from build123d import *

# Parameters (mm, degrees)
SKETCH1_W          = 127
SKETCH1_H          = 6.35
SKETCH2_R          = 6.35
CUT_EXTRUDE1_DEPTH = 4.826


with BuildPart() as part:
    # Sketch1 → Revolve1 (revolve)
    with BuildSketch(Plane.XY, mode=Mode.PRIVATE) as revolve1_sk:
        with BuildLine():
            Line((127, 0), (127, 6.35))
            ThreePointArc((127, 6.35), (135.980256121, 10.069743879), (139.7, 19.05))
            Line((139.7, 19.05), (146.05, 19.05))
            ThreePointArc((146.05, 19.05), (140.470384182, 5.579615818), (127, 0))
        make_face()
        with Locations((63.5, 3.175)):
            Rectangle(SKETCH1_W, SKETCH1_H)
    revolve(revolve1_sk.sketch.rotate(Axis((0, 0, 0), (0, 1, 0)), 90), axis=Axis((0, 0, 0), (0, 1, 0)))

    # Sketch2 → Cut-Extrude1 (cut)
    with BuildSketch(Plane.XZ):
        with Locations(Location((0, 0, 0), (0, 0, 270))):
            Circle(SKETCH2_R)
    extrude(amount=-CUT_EXTRUDE1_DEPTH, mode=Mode.SUBTRACT)


solid = part.part
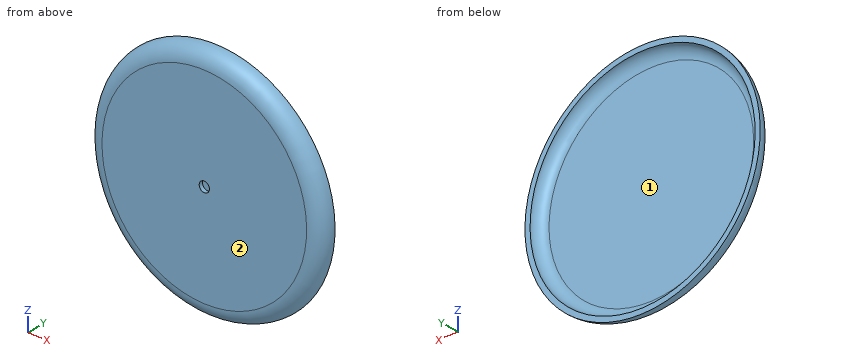
Part model, mm, in its own coordinate system. Face numbers are marked on the shaded views. Coordinates: 2 decimals unless noted, no trailing zeros. Order: outer loops, then holes, each group sorted by start corner. A loop starts at its lowest first (then second) coordinate and runs counter-clockwise, first axis right, second up. Notation, with made-up numbers: M 4.25,47 L 52.25,47 A24 cw 52.25,73 Z; hole C 54,54.5 d11. An arc over 180 degrees is marked long. One line per question, with ' | ' between items.
Q1. Slice it at C-C (y = 13.25). Give the cut face in (x, z).
A:
outline: C 0,0 d290.29; hole C 0,0 d276.6
Q2. Slice it at B-B (z = 0). Give the cut face in (x, y), and give its area (3 significant figures).
A:
outline: M -146.05,19.05 A19.05 ccw -127,0 L -6.35,0 L -6.35,4.83 L 6.35,4.83 L 6.35,0 L 127,0 A19.05 ccw 146.05,19.05 L 139.7,19.05 A12.7 cw 127,6.35 L -127,6.35 A12.7 cw -139.7,19.05 Z | area: 1,870 mm^2
Q3. Two-plate mould, pull along Z, no slides. Class the marked faces 1 and 2: +Z half, -Z half, draft (parallel to the pull), parting line (faces both ways), or undercut.
A:
face 1: undercut | face 2: draft
Q4. Slice it at A-A (x = 0). Give the cut face in (y, z), and give its area (3 significant figures).
A:
outline: M 0,-127 A19.05 ccw 19.05,-146.05 L 19.05,-139.7 A12.7 cw 6.35,-127 L 6.35,127 A12.7 cw 19.05,139.7 L 19.05,146.05 A19.05 ccw 0,127 L 0,6.35 L 4.83,6.35 L 4.83,-6.35 L 0,-6.35 Z | area: 1,870 mm^2
Q5. Pin check, flat tips, straight feed: P1, Ø10, axis at y = 3.5, z = -41, coming from the +X side; P2, Ø8, axis at y = 4, z = 63.5, coming from the +X side; P3, Ø1, axis at y = 2, z = 39, coming from the -X side. Stop position of each tip, or through.
A:
P1: stops at x = 137.14 | P2: stops at x = 128.13 | P3: stops at x = -130.75
Q6. Drill centre lines: line 1 (Y direction, x = 44, z = 2.5); line 2 (X direction, y = 7.75, z = 24); line 3 (X direction, y = 1.95, z = 0). Where is each one in solid material? Low to high.
A:
line 1: y = 0 to 6.35 | line 2: x = -140.3 to -130.61, 130.61 to 140.3 | line 3: x = -135.4 to -6.35, 6.35 to 135.4
